Here's how the part is built. I have some questions about the finished solid (model axes, mm). A direction names the side the tool comes from. Coordinates: 2 decimals unless noted, no trailing zeros. Write each loop counter-clockwise with the first axis right and the second up, starting at its lowest first coordinate (ties: lowest second). Pieces come first, ordered by that corner, then holes.
```python
from build123d import *

# Parameters (mm, degrees)
SKETCH1_R                   = 6.35
BOSS_EXTRUDE1_DEPTH         = 22.07514
SKETCH2_R                   = 6.35
BOSS_EXTRUDE2_DEPTH         = 10.16
F_1_4_28_TAPPED_HOLE1_D     = 5.4102
F_1_4_28_TAPPED_HOLE1_DEPTH = 15.494
F_1_4_28_TAPPED_HOLE1_TIP   = 1.625388061
SKETCH5_R                   = 6.35
BOSS_EXTRUDE3_DEPTH         = 3.175


with BuildPart() as part:
    # Sketch1 → Boss-Extrude1 (new body)
    with BuildSketch(Plane(origin=(0, 0, 0), x_dir=(1, 0, 0), z_dir=(0, 1, 0))):
        Circle(SKETCH1_R)
    extrude(amount=BOSS_EXTRUDE1_DEPTH)

    # Sketch2 → Boss-Extrude2 (add)
    with BuildSketch(Plane.XZ):
        Circle(SKETCH2_R)
    extrude(amount=BOSS_EXTRUDE2_DEPTH)

    # 1/4-28 Tapped Hole1
    with Locations(Plane(origin=(0, -10.16, 0), x_dir=(-1, 0, 0), z_dir=(0, -1, 0))):
        with Locations((0, 0)):
            Hole(F_1_4_28_TAPPED_HOLE1_D / 2, depth=F_1_4_28_TAPPED_HOLE1_DEPTH)
            with Locations((0, 0, -(F_1_4_28_TAPPED_HOLE1_DEPTH + F_1_4_28_TAPPED_HOLE1_TIP / 2))):  # 118° drill point
                Cone(0, F_1_4_28_TAPPED_HOLE1_D / 2, F_1_4_28_TAPPED_HOLE1_TIP, mode=Mode.SUBTRACT)

    # Sketch5 → Boss-Extrude3 (add)
    with BuildSketch(Plane(origin=(0, 22.07514, 0), x_dir=(1, 0, 0), z_dir=(0, 1, 0))):
        Circle(SKETCH5_R)
    extrude(amount=-BOSS_EXTRUDE3_DEPTH)


solid = part.part
```
1) Imagine slicing it at C-C on z = -4. Please give me the cut outline in (x, y), then the cut area to 3 significant figures.
Values follow:
outline: (-4.93, -10.16) - (4.93, -10.16) - (4.93, 22.08) - (-4.93, 22.08) - close
area: 318 mm2
2) Will these pins go through, and if not, where does the flat tip stop? pin 1 (3 mm diameter, centred on x = 4, y = 3, fed in from +Z); pin 2 (1.5 mm diameter, centred on y = 7, z = -1.5, fed in from -X); pin 3 (7 mm diameter, centred on x = 0, z = 0, fed in from -Y); pin 4 (2 mm diameter, centred on x = 4.5, y = 5, fed in from -Z).
Values follow:
pin 1: stops at z = 5.84
pin 2: stops at x = -6.31
pin 3: stops at y = -10.16
pin 4: stops at z = -5.3
3) Imagine slicing it at A-A on y = 0. Please give me the cut outline in (x, z), then the cut area to 3 significant figures.
Values follow:
outline: circle Ø12.7 at (0, 0); hole circle Ø5.41 at (0, 0)
area: 104 mm2
4) On a 3-axis mill with a long thin cutter (end or side, diameter ignored), from which of +Z, -Z, +X, -X, +Y, -Y can I reach the whole of each face in a straight line? I mean faces 1 (the face through (2.58, -2.3, -0.81)), 2 (the face through (3, -10.16, 0)). Say none if no direction works.
Values follow:
face 1: -Y
face 2: +Z, -Z, +X, -X, -Y
5) Imagine slicing it at B-B on x = 5.75. Please give me the cut outline in (y, z).
Values follow:
outline: (-10.16, -2.69) - (22.08, -2.69) - (22.08, 2.69) - (-10.16, 2.69) - close
6) I need wall thicknesses on probe 1 along Z at (x, y) = (0, 1.25); probe 2 along X at (y, z) = (-7, 0.5); probe 3 along X at (y, z) = (-5.5, 5.25). Which ranges of each line are inside material? Lowest first, please.
Values follow:
probe 1: z = -6.35 to -2.71, 2.71 to 6.35
probe 2: x = -6.33 to -2.66, 2.66 to 6.33
probe 3: x = -3.57 to 3.57
7) We'd pull the mould along Z, two halves only. Please class faces 3 (the face through (-1.38, 6.18, -6.2)), 4 (the face through (-0.448, 6.677, -0.141)), 5 (the face through (0, 22.075, 0)): pulls with the +Z half, pulls with the -Z half, needs draft (parallel to the pull), parting line crosses it, or undercut.
Values follow:
face 3: parting line crosses it
face 4: undercut
face 5: needs draft
